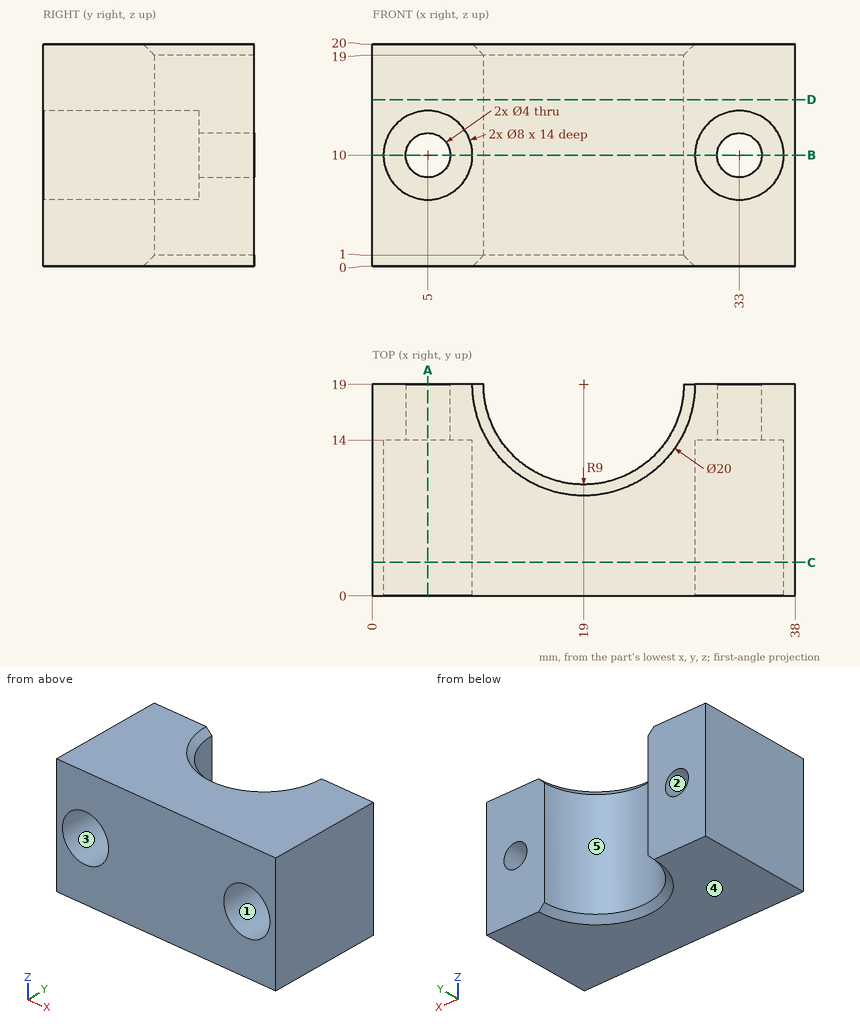
The drawing under review shows one solid part. Ordinate dimensions are in mm from its lowest x, y, z. A direction names the side the tool comes from. Round coordinates to 2 decimals unless told otherwise and drop trailing zeros. Loops run counter-clockwise (first coordinate to the right, second up) from the corner with the lowest first, then second, coordinate; pieces in that order, holes last. Notation, with made-up numbers: (-8, 78) - (-3, 78) arc R23 cw to (-3, 90) - close; hole circle Ø6 at (-4, -5.5). An arc over 180 degrees is marked (long way). One line per question, with ' | ' between items.
1. We need section C-C, the plane y = 3. State the section outline as (x, z) points.
Results are:
outline: (0, 0) - (38, 0) - (38, 20) - (0, 20) - close; hole circle Ø8 at (5, 10); hole circle Ø8 at (33, 10)
2. For L1, parallel to Z at x = 33, y = 10; L2, parallel to Z at x = 5, y = 17.1; L3, parallel to X at y = 4, z = 9, list the stretches that pass through material, from the lowest coordinate up. Write a range as [from, to].
Results are:
L1: z = [0, 6], [14, 20] | L2: z = [0, 8], [12, 20] | L3: x = [0, 1.13], [8.87, 29.13], [36.87, 38]
3. We need section D-D, the plane z = 15. State the section outline as (x, y) points, and give its area (3 significant figures).
Results are:
outline: (0, 0) - (38, 0) - (38, 19) - (28, 19) arc R9 cw to (10, 19) - (0, 19) - close | area: 595 mm²
4. We need section B-B, the plane z = 10. State the section outline as (x, y) points.
Results are:
outline: (0, 0) - (1, 0) - (1, 14) - (3, 14) - (3, 19) - (0, 19) - close; (7, 14) - (9, 14) - (9, 0) - (29, 0) - (29, 14) - (31, 14) - (31, 19) - (28, 19) arc R9 cw to (10, 19) - (7, 19) - close; (35, 14) - (37, 14) - (37, 0) - (38, 0) - (38, 19) - (35, 19) - close
5. We need section A-A, the plane x = 5. State the section outline as (y, z) points.
Results are:
outline: (0, 0) - (19, 0) - (19, 8) - (14, 8) - (14, 6) - (0, 6) - close; (0, 14) - (14, 14) - (14, 12) - (19, 12) - (19, 20) - (0, 20) - close
6. For the marked faces 1 and 2, list the 3-axis set-ups (+Z, -Z, +X, -X, +Y, -Y) from which the entire face can be reached by the end or side of a thin tool; tool diameter is ignored.
Results are:
face 1: -Y | face 2: +Y, -Y
7. Draft analysis for pull direction Z (two halves, no side actions). For the marked faces 3, 4 and 5, state which applies: released by +Z, released by -Z, zero draft, split by the parting line, or undercut.
Results are:
face 3: undercut | face 4: released by -Z | face 5: zero draft
